For this review, take the finished solid that the model builds, in its own axes (mm). A direction names the side the tool comes from. Coordinates: 2 decimals unless noted, no trailing zeros. Write each loop counter-clockwise with the first axis right and the second up, starting at its lowest first coordinate (ties: lowest second). Pieces come first, ordered by that corner, then holes.
```python
from build123d import *

# Parameters (mm, degrees)
BOSS_EXTRUDE1_DEPTH = 6.35
CUT_EXTRUDE1_DEPTH  = 300.596203247
SKETCH4_W           = 6.35
SKETCH4_H           = 81.28
SKETCH4_H_2         = 63.5
BOSS_EXTRUDE3_DEPTH = 6.35
SKETCH5_R           = 1.4732
CUT_EXTRUDE2_DEPTH  = 300.596203247
SKETCH6_R           = 3.175
SKETCH6_R_2         = 3.174999999
SKETCH6_R_3         = 1.4732
CUT_EXTRUDE3_DEPTH  = 300.596203247
CUT_EXTRUDE4_REACH  = 301.596
SKETCH7_R           = 3.1763843
SKETCH8_R           = 1.4605
CUT_EXTRUDE5_DEPTH  = 300.596203247
SKETCH11_R          = 20.574
CUT_EXTRUDE6_DEPTH  = 25.4


with BuildPart() as part:
    # Sketch1 → Boss-Extrude1 (new body)
    with BuildSketch(Plane(origin=(0, 0, 0), x_dir=(0, 0, -1), z_dir=(1, 0, 0))):
        Polygon((63.5, 158.75), (139.7, 158.75), (190.5, 158.75), (190.5, 152.4), (254, 152.4), (254, 107.95), (139.7, 107.95), (139.7, 0), (0, 0), (0, 152.4), (63.5, 152.4), align=None)
    extrude(amount=BOSS_EXTRUDE1_DEPTH)

    # Sketch2 → Cut-Extrude1 (cut, through all)
    with BuildSketch(Plane.ZY):
        Polygon((0, 17.526), (-3.96875, 17.526), (-3.96875, 15.8242), (-6.35, 15.8242), (-6.35, 17.526), (-12.7, 17.526), (-12.7, 20.4724), (-6.35, 20.4724), (-6.35, 22.1742), (-3.96875, 22.1742), (-3.96875, 20.4724), (0, 20.4724), align=None)
        Polygon((-139.7, 17.526), (-139.7, 20.4724), (-135.73125, 20.4724), (-135.73125, 22.1742), (-133.35, 22.1742), (-133.35, 20.4724), (-127, 20.4724), (-127, 17.526), (-133.35, 17.526), (-133.35, 15.8242), (-135.73125, 15.8242), (-135.73125, 17.526), align=None)
        Polygon((-12.7, 134.7724), (-12.7, 131.826), (-6.35, 131.826), (-6.35, 130.1242), (-3.96875, 130.1242), (-3.96875, 131.826), (0, 131.826), (0, 134.7724), (-3.96875, 134.7724), (-3.96875, 136.4742), (-6.35, 136.4742), (-6.35, 134.7724), align=None)
    extrude(amount=-CUT_EXTRUDE1_DEPTH, mode=Mode.SUBTRACT)

    # Sketch4 → Boss-Extrude3 (add)
    with BuildSketch(Plane.ZY):
        with Locations((3.175, 76.2)):
            Rectangle(SKETCH4_W, SKETCH4_H)
        with Locations((-142.875, 76.2)):
            Rectangle(SKETCH4_W, SKETCH4_H_2)
    extrude(amount=-BOSS_EXTRUDE3_DEPTH)

    # Sketch5 → Cut-Extrude2 (cut, through all)
    with BuildSketch(Plane.ZY):
        with Locations(Location((3.175, 41.91, 0), (0, 0, 180))):
            Circle(SKETCH5_R)
        with Locations((-142.875, 76.2)):
            Circle(SKETCH5_R)
        with Locations((3.175, 110.49)):
            Circle(SKETCH5_R)
    extrude(amount=-CUT_EXTRUDE2_DEPTH, mode=Mode.SUBTRACT)

    # Sketch6 → Cut-Extrude3 (cut, through all)
    with BuildSketch(Plane.ZY):
        with Locations((-61.214, 136.503809763)):
            Circle(SKETCH6_R)
        with Locations((-80.009999999, 133.35)):
            Circle(SKETCH6_R_2)
        with Locations((-95.25, 155.575)):
            Circle(SKETCH6_R_3)
        with Locations((-158.75, 155.575)):
            Circle(SKETCH6_R_3)
        with Locations((-188.224, 136.50380976)):
            Circle(SKETCH6_R)
        with Locations((-173.99, 133.35)):
            Circle(SKETCH6_R)
        with Locations((-124.719, 148.476804798)):
            Circle(SKETCH6_R)
        with Locations((-124.719, 121.898809762)):
            Circle(SKETCH6_R)
        Polygon((-30.2641, 152.4), (-33.2105, 152.4), (-33.2105, 148.59), (-35.0393, 148.59), (-35.0393, 146.05), (-33.2105, 146.05), (-33.2105, 139.7), (-30.2641, 139.7), (-30.2641, 146.05), (-28.4353, 146.05), (-28.4353, 148.59), (-30.2641, 148.59), align=None)
        Polygon((-220.7895, 152.4), (-223.7359, 152.4), (-223.7359, 148.59), (-225.5647, 148.59), (-225.5647, 146.05), (-223.7359, 146.05), (-223.7359, 139.7), (-220.7895, 139.7), (-220.7895, 146.05), (-218.9607, 146.05), (-218.9607, 148.59), (-220.7895, 148.59), align=None)
    extrude(amount=-CUT_EXTRUDE3_DEPTH, mode=Mode.SUBTRACT)

    # Sketch7 → Cut-Extrude4 (cut, up to next)
    with BuildSketch(Plane(origin=(6.35, 0, 0), x_dir=(0, 0, -1), z_dir=(1, 0, 0)), mode=Mode.PRIVATE) as cut_extrude4_sk1:
        with Locations((-1.419543332, 94.061078275)):
            Circle(SKETCH7_R)
    cut_extrude4_tool1 = extrude(cut_extrude4_sk1.sketch, amount=-CUT_EXTRUDE4_REACH, mode=Mode.PRIVATE) & part.part
    add(cut_extrude4_tool1.solids().sort_by_distance((6.35, 94.061078, 1.419543))[0], mode=Mode.SUBTRACT)

    # Sketch8 → Cut-Extrude5 (cut, through all)
    with BuildSketch(Plane.ZY):
        with Locations((-171.45, 114.3)):
            Circle(SKETCH8_R)
        with Locations((-171.45, 139.7)):
            Circle(SKETCH8_R)
    extrude(amount=-CUT_EXTRUDE5_DEPTH, mode=Mode.SUBTRACT)

    # Sketch11 → Cut-Extrude6 (cut)
    with BuildSketch(Plane.ZY):
        with Locations((-22.86, 114.3)):
            Circle(SKETCH11_R)
    extrude(amount=-CUT_EXTRUDE6_DEPTH, mode=Mode.SUBTRACT)


solid = part.part
```
Q1. Add section A-A (z = -39). State the section outline as (x, y) points.
Ans:
outline: (0, 0) - (6.35, 0) - (6.35, 101.54) - (0, 101.54) - close; (0, 127.06) - (6.35, 127.06) - (6.35, 152.4) - (0, 152.4) - close
Q2. Add section D-D (z = -213). State the section outline as (x, y) points.
Ans:
outline: (0, 107.95) - (6.35, 107.95) - (6.35, 152.4) - (0, 152.4) - close
Q3. Draft analysis for pull direction Y (two halves, no side actions). For faces 1 (the flat face through (3, 116.84, 3)), 2 (the cylindrical face through (3.13, 139.65, -188.64)), 3 (the flat face through (3, 143, -223.736)), state which applies: +Y half, -Y half, draft (parallel to the pull), parting line (faces both ways), or undercut.
Ans:
face 1: +Y half
face 2: undercut
face 3: draft
Q4. Add section B-B (y = 12.5). State the section outline as (x, z) points.
Ans:
outline: (0, -139.7) - (6.35, -139.7) - (6.35, 0) - (0, 0) - close
Q5. Clearance check with flat-ended pins moving along their axes: pin 1 Ø1.9 at (x, z) = (2.5, -143.5) entering from -Y; pin 2 Ø3 at (x, z) = (3.5, -50) entering from +Y; pin 3 Ø3 at (x, y) = (2.5, 134) entering from +Z. State where each tip first meets the part, or that it passes through.
Ans:
pin 1: stops at y = 44.45
pin 2: stops at y = 152.4
pin 3: stops at z = 0
Q6. Tool access review of faces 4 (the flat face through (3, 9, 0)), 5 (the flat face through (3, 143, 0)), 6 (the flat face through (3, 156, -190.5)): name each direction out of +Z, -Z, +X, -X, +Y, -Y from which nothing blocks a thin tool from reaching the whole face with its end or side.
Ans:
face 4: +Z, +X, -X, -Y
face 5: +Z, +X, -X, +Y
face 6: -Z, +X, -X, +Y
Q7. For probe 1 along Z at (x, y) = (4.5, 143); probe 2 along Z at (x, y) = (3.5, 114.3); probe 3 along Y at (x, z) = (3.5, -158.75), list the stretches that pass through material, from the lowest coordinate up.
Ans:
probe 1: z = -254 to -223.74, -220.79 to -33.21, -30.26 to 0
probe 2: z = -254 to -172.91, -169.99 to -43.43, -2.29 to 6.35
probe 3: y = 107.95 to 154.1, 157.05 to 158.75
Q8. Add section C-C (x = 1.5). Give the number of separate pieces and of enclosed holes in the cut face, then the cut area to 3 significant figures.
Ans:
separate pieces: 1
enclosed holes: 14
area: 26,300 mm2
